The listing builds one solid part. Answer for the finished solid, in the listing's coordinates (mm). Give positions to 0.01 mm unless a question says otherwise; leave off trailing zeros. Loops run counter-clockwise (first coordinate to the right, second up) from the corner with the lowest first, then second, coordinate; pieces in that order, holes last.
Item 1: Section A-A, the plane z = 9.75 is taken. Give the vertices of the cut face in (x, y).
Item 2: Section B-B, the plane y = -10.5 is taken. Give the vertices of the cut face in (x, z).
Item 3: Section C-C, the plane z = 6 is taken. Give the vertices of the cut face in (x, y), and give its area (3 significant figures).
Item 4: Consider line 1 along X through (y, z) = (-6, 4); line 2 along X through (y, z) = (-4.5, 6.25). Determine where each line is inside the solid, lowest interval first.
Item 5: This flat-tipped pin is pushed along its axis until it touches: pin 1 Ø4 at (y, z) = (-11.5, 7.5) entering from +X. Where does it stop, or does it pass through?
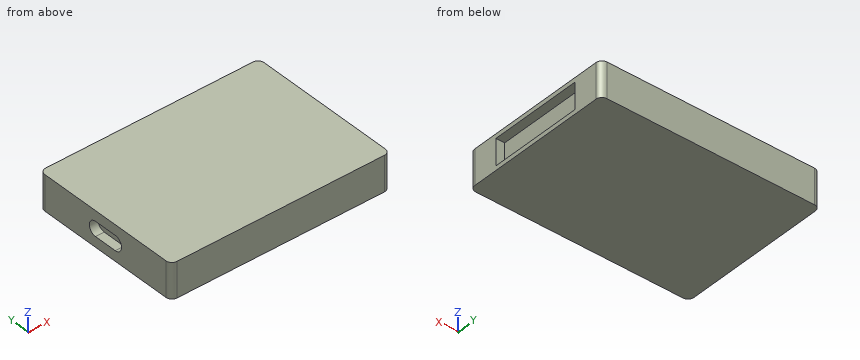
from build123d import *

# Parameters (mm, degrees)
SKETCH_1_W          = 75
SKETCH_1_H          = 53
EXTRUDE_1_DEPTH     = 12
FILLET_1_R          = 2
SKETCH_2_W          = 9
SKETCH_2_H          = 32
CUT_EXTRUDE_1_DEPTH = 3
CUT_EXTRUDE_2_DEPTH = 3


with BuildPart() as part:
    # 草图1 → 凸台-拉伸1 (new body)
    with BuildSketch(Plane.XY):
        Rectangle(SKETCH_1_W, SKETCH_1_H)
    extrude(amount=EXTRUDE_1_DEPTH)

    # 圆角1
    fillet_1_edges = [part.edges().sort_by_distance(p)[0] for p in [
        (-37.5, 26.5, 6),
        (37.5, 26.5, 6),
        (37.5, -26.5, 6),
        (-37.5, -26.5, 6),
    ]]
    fillet(fillet_1_edges, radius=FILLET_1_R)

    # 草图2 → 切除-拉伸1 (cut)
    with BuildSketch(Plane(origin=(37.5, 0, 0), x_dir=(0, 0, -1), z_dir=(1, 0, 0))):
        with Locations((-6, 0)):
            Rectangle(SKETCH_2_W, SKETCH_2_H)
    extrude(amount=-CUT_EXTRUDE_1_DEPTH, mode=Mode.SUBTRACT)

    # 草图3 → 切除-拉伸2 (cut)
    with BuildSketch(Plane.ZY.offset(37.5)):
        with BuildLine():
            Line((3.5, -4), (3.5, 4))
            ThreePointArc((3.5, 4), (6, 6.5), (8.5, 4))
            Line((8.5, 4), (8.5, -4))
            ThreePointArc((8.5, -4), (6, -6.5), (3.5, -4))
        make_face()
    extrude(amount=-CUT_EXTRUDE_2_DEPTH, mode=Mode.SUBTRACT)


solid = part.part
Worked answers:
1. outline: (-37.5, -24.5) arc R2 ccw to (-35.5, -26.5) - (35.5, -26.5) arc R2 ccw to (37.5, -24.5) - (37.5, -16) - (34.5, -16) - (34.5, 16) - (37.5, 16) - (37.5, 24.5) arc R2 ccw to (35.5, 26.5) - (-35.5, 26.5) arc R2 ccw to (-37.5, 24.5) - close
2. outline: (-37.5, 0) - (37.5, 0) - (37.5, 1.5) - (34.5, 1.5) - (34.5, 10.5) - (37.5, 10.5) - (37.5, 12) - (-37.5, 12) - close
3. outline: (-37.5, -24.5) arc R2 ccw to (-35.5, -26.5) - (35.5, -26.5) arc R2 ccw to (37.5, -24.5) - (37.5, -16) - (34.5, -16) - (34.5, 16) - (37.5, 16) - (37.5, 24.5) arc R2 ccw to (35.5, 26.5) - (-35.5, 26.5) arc R2 ccw to (-37.5, 24.5) - (-37.5, 6.5) - (-34.5, 6.5) - (-34.5, -6.5) - (-37.5, -6.5) - close
3. area: 3,840 mm2
4. line 1: x = -37.5 to 34.5
4. line 2: x = -34.5 to 34.5
5. pin 1: stops at x = 34.5
